Check sheet for the drawn part. Datum: minimum x, y, z corner. Units: mm. A direction names the side the tool comes from. Coordinates: 2 decimals unless noted, no trailing zeros. Write each loop counter-clockwise with the first axis right and the second up, starting at its lowest first coordinate (ties: lowest second). Pieces come first, ordered by that corner, then holes. Notation, with made-up numbers: (-37.5, -12.75) -> (-30.5, -12.75) arc R12 ccw to (-30.5, 7.25) -> close; hole circle Ø1 at (-6.5, 89). An arc over 180 degrees is marked (long way). Answer in a Markdown table with one row per item.
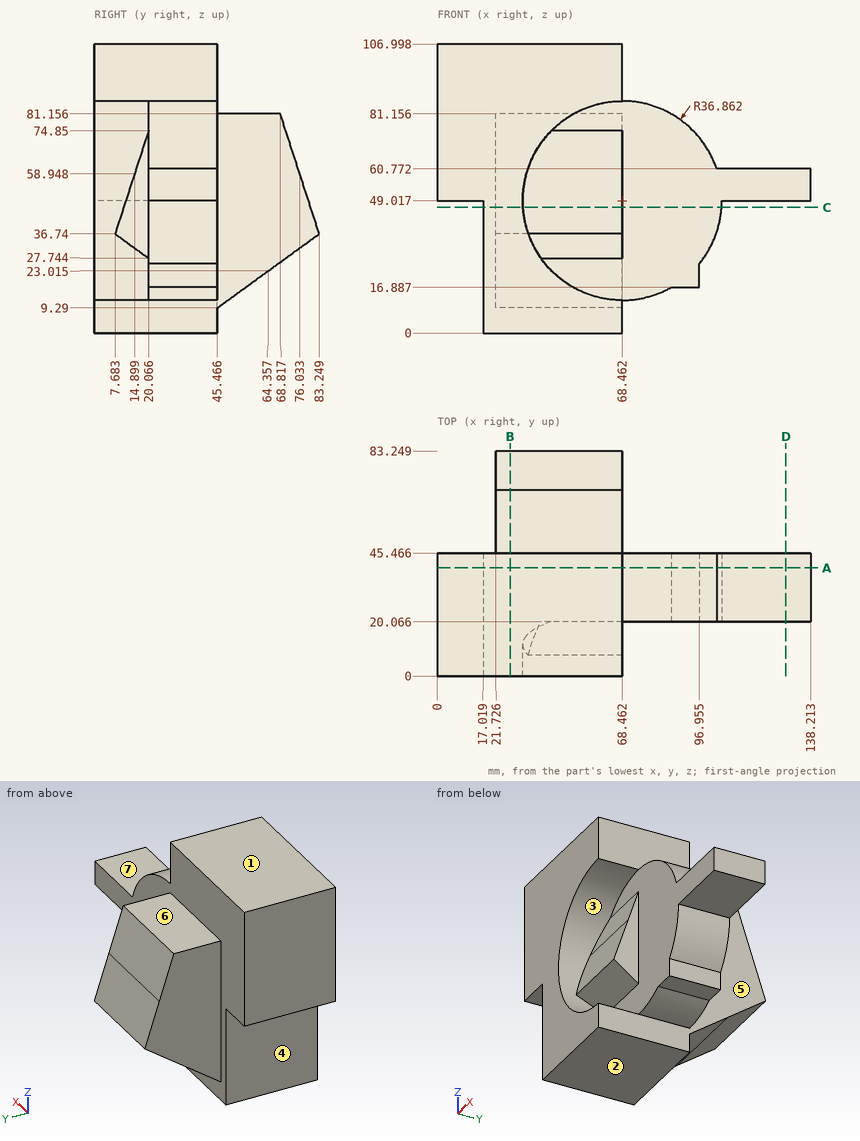
1. Go/stop test with flat-tipped pins: pin 1 (3 mm diameter, centred on x = 94, y = 30, fed in from -Z); pin 2 (7.5 mm diameter, centred on x = 121, y = 30, fed in from -Z); pin 3 (2 mm diameter, centred on y = 74, z = 66, fed in from -X). Record where each tip stops, or that it passes through.
Findings below:
| item | result |
|---|---|
| pin 1 | stops at z = 16.89 |
| pin 2 | stops at z = 49.02 |
| pin 3 | stops at x = 21.73 |
2. Release check for a two-part mould opening along Z. For the marked faces 1, 2 and 3 record: released by +Z, released by -Z, zero draft, split by the parting line, or undercut.
Findings below:
| item | result |
|---|---|
| face 1 | released by +Z |
| face 2 | released by -Z |
| face 3 | undercut |
3. Material ranges on probe 1 along Z at (x, y) = (12, 13); probe 2 along Y at (x, z) = (36, 59) (1 decimal); probe 3 along X at (y, z) = (69, 52) (1 decimal), recorded low to high. Write a range as from..to.
Findings below:
| item | result |
|---|---|
| probe 1 | z = 49.02..107 |
| probe 2 | y = 14.9..76 |
| probe 3 | x = 21.7..68.5 |
4. Access from +Z, -Z, +X, -X, +Y, -Y to the whole of each face (thin tool, end or side, straight path). Record for the marked faces 4, 5, 6 and 7.
Findings below:
| item | result |
|---|---|
| face 4 | -Z, -X, +Y, -Y |
| face 5 | -Z, +X, +Y |
| face 6 | +Z, +X, -X, +Y |
| face 7 | +Z, +X, +Y, -Y |
5. Sectioned sample at C-C, the plane z = 46.5. Record the cut outline in (x, y) (1 decimal).
Findings below:
| item | result |
|---|---|
| outline | (17, 0) -> (31.7, 0) -> (31.7, 10.9) -> (68.5, 10.9) -> (68.5, 20.1) -> (105.2, 20.1) -> (105.2, 45.5) -> (68.5, 45.5) -> (68.5, 80.1) -> (21.7, 80.1) -> (21.7, 45.5) -> (17, 45.5) -> close |
6. Sectioned sample at B-B, the plane x = 27. Record the cut outline in (y, z) (1 decimal), and give its area (3 significant figures).
Findings below:
| item | result |
|---|---|
| outline | (0, 0) -> (45.5, 0) -> (45.5, 9.3) -> (83.2, 36.7) -> (68.8, 81.2) -> (45.5, 81.2) -> (45.5, 107) -> (0, 107) -> close |
| area | 6,740 mm² |
7. Sectioned sample at D-D, the plane x = 129. Record the cut outline in (y, z).
Findings below:
| item | result |
|---|---|
| outline | (20.07, 49.02) -> (45.47, 49.02) -> (45.47, 60.77) -> (20.07, 60.77) -> close |
8. Sectioned sample at A-A, the plane y = 40. Record the cut outline in (x, z) (1 decimal), and give its area (3 significant figures).
Findings below:
| item | result |
|---|---|
| outline | (0, 49) -> (17, 49) -> (17, 0) -> (68.5, 0) -> (68.5, 12.2) arc R36.9 ccw to (86.5, 16.9) -> (97, 16.9) -> (97, 25.6) arc R36.9 ccw to (105.3, 49) -> (138.2, 49) -> (138.2, 60.8) -> (103.4, 60.8) arc R36.9 ccw to (68.5, 85.9) -> (68.5, 107) -> (0, 107) -> close |
| area | 9,060 mm² |
